from build123d import *

# Parameters (mm, degrees)
SKETCH_1_R          = 92.5
SKETCH_1_R_2        = 15.2
EXTRUDE_1_DEPTH     = 5
SKETCH_8_W          = 5
SKETCH_8_H          = 7
EXTRUDE_2_DEPTH     = 85
SKETCH_11_R         = 1.45
CUT_EXTRUDE_1_DEPTH = 85
SKETCH_12_W         = 54
SKETCH_12_H         = 16
CUT_EXTRUDE_2_DEPTH = 85
SKETCH_14_W         = 20
SKETCH_14_H         = 10
CUT_EXTRUDE_3_DEPTH = 100


with BuildPart() as part:
    # 스케치1 → 보스-돌출1 (new body)
    with BuildSketch(Plane(origin=(0, 0, 0), x_dir=(1, 0, 0), z_dir=(0, 1, 0))):
        Circle(SKETCH_1_R)
        Circle(SKETCH_1_R_2, mode=Mode.SUBTRACT)
    extrude(amount=EXTRUDE_1_DEPTH)

    # 스케치5 → 회전1 (revolve)
    with BuildSketch(Plane.XY):
        Polygon((-92.5, 5), (-96.5, 83), (-91.5, 83), (-87.5, 5), align=None)
    revolve(axis=Axis((0, 0, 0), (0, 1, 0)))

    # 스케치8 → 회전3 (revolve)
    with BuildSketch(Plane.XY):
        with Locations((-94, 86.5)):
            Rectangle(SKETCH_8_W, SKETCH_8_H)
    revolve(axis=Axis((0, 0, 0), (0, 1, 0)))

    # 스케치9 → 보스-돌출2 (add)
    with BuildSketch(Plane(origin=(0, 5, 0), x_dir=(1, 0, 0), z_dir=(0, 1, 0))):
        Polygon((-20, -25), (20, -25), (27, -25), (27, 29), (20, 29), (20, -18), (-20, -18), (-20, 29), (-27, 29), (-27, -25), align=None)
    extrude(amount=EXTRUDE_2_DEPTH)

    # 스케치11 → 컷-돌출1 (cut)
    with BuildSketch(Plane.XY.offset(25)):
        with Locations((15, 42)):
            Circle(SKETCH_11_R)
        with Locations((-15, 42)):
            Circle(SKETCH_11_R)
        with Locations((-15, 66)):
            Circle(SKETCH_11_R)
        with Locations((15, 66)):
            Circle(SKETCH_11_R)
    extrude(amount=-CUT_EXTRUDE_1_DEPTH, mode=Mode.SUBTRACT)

    # 스케치12 → 컷-돌출2 (cut)
    with BuildSketch(Plane.XY.offset(25)):
        with Locations((0, 82)):
            Rectangle(SKETCH_12_W, SKETCH_12_H)
    extrude(amount=-CUT_EXTRUDE_2_DEPTH, mode=Mode.SUBTRACT)

    # 스케치14 → 컷-돌출3 (cut)
    with BuildSketch(Plane.XY):
        with Locations((0, 77.228887743)):
            Rectangle(SKETCH_14_W, SKETCH_14_H)
    extrude(amount=-CUT_EXTRUDE_3_DEPTH, mode=Mode.SUBTRACT)


solid = part.part
CAD build for the part. Positions are in the model's coordinates, mm. A direction names the side the tool comes from. Coordinates: 2 decimals unless noted, no trailing zeros. Loops run counter-clockwise (first coordinate to the right, second up) from the corner with the lowest first, then second, coordinate; pieces in that order, holes last. Notation, with made-up numbers: (-23.5, -14.5) - (-5.5, -14.5) arc R23 ccw to (-5.5, 0.5) - close; hole circle Ø11 at (53, -19.5). An arc over 180 degrees is marked (long way). Write item = value, one per line. Start each with the question number.
Q1. Which spindle directions (+Z, -Z, +X, -X, +Y, -Y) get a long thin tool onto all of the face, cutting with end or side? Do faces 4 (the cylindrical face through (49.727, 2.465, -77.996)), 5 (the flat face through (-1, 0, 19)), 6 (the flat face through (0, 72.229, -93)), 7 (the flat face through (-20, 39, -5)). Say none if no direction does.
Q2. Drill centre lines: L1, parallel to X at y = 2.9, z = 0; L2, parallel to X at y = 30.5, z = -9.5; L3, parallel to Z at x = 13, y = 17.5. Where is each one in solid material? Low to high.
Q3. Pull direction Y, two halves, no side cores. Call faces 1 (the flat face through (0, 39, 25)), 2 (the flat face through (0, 82.229, -94)), 3 (the conical face through (11.59, 34.79, 88.27)): pulls with the +Y half, pulls with the -Y half, needs draft (parallel to the pull), parting line crosses it, or undercut.
Q4. Cut at B-B, the plane x = 0. List the corners of the cut face in (y, z).
Q5. Flat gauge pins, fed straight in: pin 1 Ø10 at (y, z) = (44.5, 48.5) entering from -X; pin 2 Ø5.5 at (x, y) = (-22.5, 34) entering from -Z; pin 3 Ø2.5 at (x, y) = (15, 66) entering from -Z. Where does each tip first touch, or does it go through?
Q6. Cut at A-A, the plane y = 23. List the corners of the cut face in (x, z).
Q7. Cut at D-D, the plane z = 22.5. Give the number of separate pieces and of enclosed holes in the cut face, then the cut area to 3 significant figures.
Q8. Cut at C-C, the plane y = 10. List the corners of the cut face in (x, z).
Computed:
q1.face_4 = -Y
q1.face_5 = +Z, -Z, +X, -X, -Y
q1.face_6 = -Z
q1.face_7 = +Y
q2.L1 = -92.5 to -15.2, 15.2 to 92.5
q2.L2 = -93.33 to -88.3, -27 to -20, 20 to 27, 88.3 to 93.33
q2.L3 = -92.23 to -87.18, 18 to 25, 87.18 to 92.23
q3.face_1 = needs draft
q3.face_2 = undercut
q3.face_3 = pulls with the +Y half
q4.outline = (0, -92.5) - (5, -92.5) - (72.23, -95.95) - (72.23, -90.95) - (5, -87.5) - (5, -15.2) - (0, -15.2) - close; (0, 15.2) - (5, 15.2) - (5, 18) - (74, 18) - (74, 25) - (5, 25) - (5, 87.5) - (83, 91.5) - (90, 91.5) - (90, 96.5) - (83, 96.5) - (5, 92.5) - (0, 92.5) - close; (82.23, -96.46) - (83, -96.5) - (90, -96.5) - (90, -91.5) - (83, -91.5) - (82.23, -91.46) - close
q5.pin_1 = -83.94
q5.pin_2 = -91.91
q5.pin_3 = -94.65
q6.outline = circle Ø186.85 at (0, 0); (-27, -29) - (-20, -29) - (-20, 18) - (20, 18) - (20, -29) - (27, -29) - (27, 25) - (-27, 25) - close; hole circle Ø176.85 at (0, 0)
q7.separate_pieces = 1
q7.enclosed_holes = 4
q7.area = 5,470 mm²
q8.outline = circle Ø185.51 at (0, 0); (-27, -29) - (-20, -29) - (-20, 18) - (20, 18) - (20, -29) - (27, -29) - (27, 25) - (-27, 25) - close; hole circle Ø175.51 at (0, 0)
